Input: dimensioned drawing with shaded views. Units: mm. Origin: part minimum x, y, z. A direction names the side the tool comes from. Give positions to 0.01 mm unless a question says otherwise; leave off trailing zeros. Loops run counter-clockwise (first coordinate to the right, second up) from the corner with the lowest first, then second, coordinate; pieces in that order, holes last.
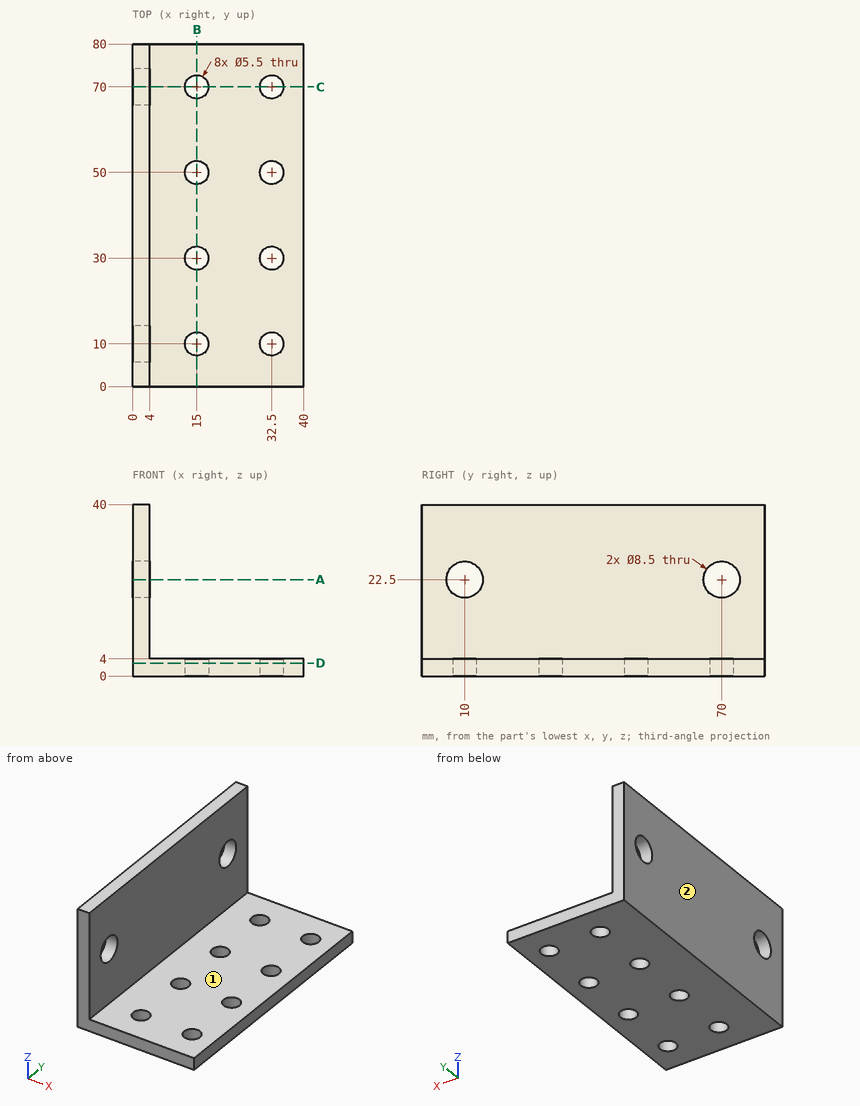
(1) First-contact query: pin 1 (4.5 mm diameter, centred on x = 32.5, y = 50, fed in from +Z); pin 2 (3 mm diameter, centred on y = 11, z = 34, fed in from +X); pin 3 (6 mm diameter, centred on x = 5.5, z = 28.5, fed in from -Y); pin 4 (3 mm diameter, centred on x = 30, y = 55, fed in from +Z). Flat tips, straight axial feed; report the tip coordinate or a pass-through.
A:
pin 1: passes through
pin 2: stops at x = 4
pin 3: stops at y = 0
pin 4: stops at z = 4
(2) Section B-B, the plane x = 15. Return the cut outline in (y, z).
A:
outline: (0, 0) - (7.25, 0) - (7.25, 4) - (0, 4) - close; (12.75, 0) - (27.25, 0) - (27.25, 4) - (12.75, 4) - close; (32.75, 0) - (47.25, 0) - (47.25, 4) - (32.75, 4) - close; (52.75, 0) - (67.25, 0) - (67.25, 4) - (52.75, 4) - close; (72.75, 0) - (80, 0) - (80, 4) - (72.75, 4) - close
(3) Section A-A, the plane z = 22.5. Return the cut outline in (x, y), then the cut area to 3 significant figures.
A:
outline: (0, 0) - (4, 0) - (4, 5.75) - (0, 5.75) - close; (0, 14.25) - (4, 14.25) - (4, 65.75) - (0, 65.75) - close; (0, 74.25) - (4, 74.25) - (4, 80) - (0, 80) - close
area: 252 mm2
(4) Ray query, line 1 along Y through (x, z) = (15, 1.25); line 2 along X through (y, z) = (56, 15). Return the intervals inside material, ascending.
A:
line 1: y = 0 to 7.25, 12.75 to 27.25, 32.75 to 47.25, 52.75 to 67.25, 72.75 to 80
line 2: x = 0 to 4
(5) Reachability of the marked faces 1 and 2 from +Z, -Z, +X, -X, +Y, -Y: full face, straight path, thin tool, end or side. Return the list, or none.
A:
face 1: +Z, +X, +Y, -Y
face 2: +Z, -Z, -X, +Y, -Y
(6) Section D-D, the plane z = 3. Count the separate pieces of the cut face and the enclosed holes in it, then the cut area to 3 significant figures.
A:
separate pieces: 1
enclosed holes: 8
area: 3,010 mm2
(7) Section C-C, the plane y = 70. Return the cut outline in (x, z).
A:
outline: (0, 0) - (12.25, 0) - (12.25, 4) - (4, 4) - (4, 18.25) - (0, 18.25) - close; (0, 26.75) - (4, 26.75) - (4, 40) - (0, 40) - close; (17.75, 0) - (29.75, 0) - (29.75, 4) - (17.75, 4) - close; (35.25, 0) - (40, 0) - (40, 4) - (35.25, 4) - close
